```python
from build123d import *

# Parameters (mm, degrees)
F0_W     = 95.25
F0_H     = 46.99
F1_DEPTH = 2.54
F2_W     = 88.9
F2_H     = 46.99
F3_DEPTH = 1.27
F4_W     = 88.9
F4_H     = 46.99
F5_DEPTH = 2.54


with BuildPart() as f1:
    # F0 (on Right) → F1 (new body)
    with BuildSketch(Plane.YZ):
        Rectangle(F0_W, F0_H)
        Polygon((-0.635, 2.159), (-0.635, -14.351), (-17.145, -14.351), (-17.145, -11.811), (-24.765, -11.811), (-24.765, -9.271), (-32.385, -9.271), (-32.385, -6.731), (-40.005, -6.731), (-40.005, 9.779), (-23.495, 9.779), (-23.495, 7.239), (-15.875, 7.239), (-15.875, 4.699), (-8.255, 4.699), (-8.255, 2.159), align=None, mode=Mode.SUBTRACT)
    extrude(amount=F1_DEPTH)

    # F2 (on face) → F3 (join)
    with BuildSketch(Plane(origin=(0, 0, 0), x_dir=(0, -1, 0), z_dir=(-1, 0, 0))):
        Rectangle(F2_W, F2_H)
        Polygon((0.635, 2.159), (8.255, 2.159), (8.255, 4.699), (15.875, 4.699), (15.875, 7.239), (23.495, 7.239), (23.495, 9.779), (40.005, 9.779), (40.005, -6.731), (32.385, -6.731), (32.385, -9.271), (24.765, -9.271), (24.765, -11.811), (17.145, -11.811), (17.145, -14.351), (0.635, -14.351), align=None, mode=Mode.SUBTRACT)
        Polygon((8.255, 4.699), (8.255, 2.159), (0.635, 2.159), (0.635, -14.351), (17.145, -14.351), (17.145, -11.811), (24.765, -11.811), (24.765, -9.271), (32.385, -9.271), (32.385, -6.731), (40.005, -6.731), (40.005, 9.779), (23.495, 9.779), (23.495, 7.239), (15.875, 7.239), (15.875, 4.699), align=None)
    extrude(amount=F3_DEPTH)

    # F4 (on face) → F5 (join)
    with BuildSketch(Plane.YZ.offset(2.54)):
        Rectangle(F4_W, F4_H)
        Polygon((-15.875, 4.699), (-8.255, 4.699), (-8.255, 2.159), (-0.635, 2.159), (-0.635, -14.351), (-17.145, -14.351), (-17.145, -11.811), (-24.765, -11.811), (-24.765, -9.271), (-32.385, -9.271), (-32.385, -6.731), (-40.005, -6.731), (-40.005, 9.779), (-23.495, 9.779), (-23.495, 7.239), (-15.875, 7.239), align=None, mode=Mode.SUBTRACT)
    extrude(amount=F5_DEPTH)


solid = f1.part
```
The model under review builds one solid part; all positions refer to its coordinate system, in mm. A direction names the side the tool comes from. Coordinates: 2 decimals unless noted, no trailing zeros. Write each loop counter-clockwise with the first axis right and the second up, starting at its lowest first coordinate (ties: lowest second). Pieces come first, ordered by that corner, then holes.
1) The part is to be moulded in two halves that separate along Y. For faces 1 (the face through (4, 44.45, 0)), 2 (the face through (3, -40.005, 1)), 3 (the face through (1, -47.625, 0)), 4 (the face through (2, -1, 23.495)), say which applies: pulls with the +Y half, pulls with the -Y half, needs draft (parallel to the pull), parting line crosses it, or undercut.
2) We need section B-B on y = -9.5. State the section outline as (x, z) points (3 decimals), then the cut area to 3 significant figures.
3) To check wall thickness, follow probe 1 along Z at (x, y) = (2.25, -9) (3 decimals); probe 2 along Y at (x, z) = (0.75, 9.5) (3 decimals); probe 3 along Y at (x, z) = (2, -13) (3 decimals). State the ranges of each line that lie inside material, in increasing order.
4) We need section A-A on z = 14. State the section outline as (x, y) points (3 decimals), then the cut area to 3 significant figures.
5) Machinability: for faces 5 (the face through (0, 46, 0)), 6 (the face through (2.54, 46, 0)), 7 (the face through (0, -46, 0)), 8 (the face through (3, -8.255, 3)), which of the approach directions +Z, -Z, +X, -X, +Y, -Y give a long, thin tool a straight path to every point of the face, cutting with its end or side? Answer none if there is none.
6) Clearance check with flat-ended pins moving along their axes: pin 1 Ø1 at (y, z) = (-46, -1) entering from +X; pin 2 Ø2 at (x, z) = (4, 2) entering from -Y; pin 3 Ø1.6 at (y, z) = (46.5, 3.5) entering from -X. State where each tip first meets the part, or that it passes through.
7) We need section C-C on z = -0.5. State the section outline as (x, y) points (3 decimals), then the cut area to 3 significant figures.
Answer list:
1. face 1: pulls with the +Y half
1. face 2: undercut
1. face 3: pulls with the -Y half
1. face 4: needs draft
2. outline: (-1.27, -23.495) - (5.08, -23.495) - (5.08, -14.351) - (0, -14.351) - (0, 4.699) - (5.08, 4.699) - (5.08, 23.495) - (-1.27, 23.495) - close
2. area: 202 mm2
3. probe 1: z = -23.495 to -14.351, 4.699 to 23.495
3. probe 2: y = -47.625 to -40.005, -23.495 to 47.625
3. probe 3: y = -47.625 to -17.145, -0.635 to 47.625
4. outline: (-1.27, -44.45) - (0, -44.45) - (0, -47.625) - (2.54, -47.625) - (2.54, -44.45) - (5.08, -44.45) - (5.08, 44.45) - (2.54, 44.45) - (2.54, 47.625) - (0, 47.625) - (0, 44.45) - (-1.27, 44.45) - close
4. area: 581 mm2
5. face 5: +Z, -Z, -X, +Y
5. face 6: +Z, -Z, +X, +Y
5. face 7: +Z, -Z, -X, -Y
5. face 8: +X
6. pin 1: stops at x = 2.54
6. pin 2: stops at y = -44.45
6. pin 3: stops at x = 0
7. outline: (-1.27, -44.45) - (0, -44.45) - (0, -47.625) - (2.54, -47.625) - (2.54, -44.45) - (5.08, -44.45) - (5.08, -40.005) - (0, -40.005) - (0, -0.635) - (5.08, -0.635) - (5.08, 44.45) - (2.54, 44.45) - (2.54, 47.625) - (0, 47.625) - (0, 44.45) - (-1.27, 44.45) - close
7. area: 381 mm2
